from build123d import *

# Parameters (mm, degrees)
F0_R     = 2.5
F2_DEPTH = 492


with BuildPart() as f2:
    # F0 (on Front) → F2 (new body)
    with BuildSketch(Plane.XZ):
        with BuildLine():
            Line((6.5, 0), (2, 0))
            ThreePointArc((2, 0), (0.5857864376, -0.5857864376), (0, -2))
            Line((0, -2), (0, -6.4857100192))
            Line((0, -6.4857100192), (0.4948230833, -6.489995392))
            Line((0.4948230833, -6.489995392), (0.4948230833, -7))
            Line((0.4948230833, -7), (2, -7))
            Line((2, -7), (2, -3.0833937817))
            Line((2, -3.0833937817), (6.2, -7.2637052917))
            Line((6.2, -7.2637052917), (6.2, -12.7393398282))
            Line((6.2, -12.7393398282), (2, -16.9393398282))
            Line((2, -16.9393398282), (2, -13))
            Line((2, -13), (0.5, -13))
            Line((0.5, -13), (0.5, -13.5))
            Line((0.5, -13.5), (0, -13.5))
            Line((0, -13.5), (0, -26.4857100192))
            Line((0, -26.4857100192), (0.4948230833, -26.489995392))
            Line((0.4948230833, -26.489995392), (0.4948230833, -27))
            Line((0.4948230833, -27), (2, -27))
            Line((2, -27), (2, -23.0833937817))
            Line((2, -23.0833937817), (6.2, -27.2637052917))
            Line((6.2, -27.2637052917), (6.2, -32.7393398282))
            Line((6.2, -32.7393398282), (2, -36.9393398282))
            Line((2, -36.9393398282), (2, -33))
            Line((2, -33), (0.5, -33))
            Line((0.5, -33), (0.5, -33.5))
            Line((0.5, -33.5), (0, -33.5))
            Line((0, -33.5), (0, -38))
            ThreePointArc((0, -38), (0.5857864376, -39.4142135624), (2, -40))
            Line((2, -40), (6.5, -40))
            Line((6.5, -40), (6.5, -39.5))
            Line((6.5, -39.5), (7, -39.5))
            Line((7, -39.5), (7, -38))
            Line((7, -38), (3.0606601718, -38))
            Line((3.0606601718, -38), (7.2606601718, -33.8))
            Line((7.2606601718, -33.8), (12.7393398282, -33.8))
            Line((12.7393398282, -33.8), (16.9393398282, -38))
            Line((16.9393398282, -38), (13.015800612, -38))
            Line((13.015800612, -38), (13.015800612, -39.5))
            Line((13.015800612, -39.5), (13.5, -39.5))
            Line((13.5, -39.5), (13.5, -40))
            Line((13.5, -40), (18, -40))
            ThreePointArc((18, -40), (19.4142135624, -39.4142135624), (20, -38))
            Line((20, -38), (20, -33.4626608249))
            Line((20, -33.4626608249), (19.5363645284, -33.4624647606))
            Line((19.5363645284, -33.4624647606), (19.532302618, -32.9822008219))
            Line((19.532302618, -32.9822008219), (18, -32.9822008219))
            Line((18, -32.9822008219), (17.9998106987, -36.9393398192))
            Line((17.9998106987, -36.9393398192), (13.8264202785, -32.765949399))
            Line((13.8264202785, -32.765949399), (13.8264202785, -27.246708479))
            Line((13.8264202785, -27.246708479), (17.9998106987, -23.0606601627))
            Line((17.9998106987, -23.0606601627), (17.9998106987, -26.9999999909))
            Line((17.9998106987, -26.9999999909), (19.4998106987, -26.9999999909))
            Line((19.4998106987, -26.9999999909), (19.4998106987, -26.4999999909))
            Line((19.4998106987, -26.4999999909), (20, -26.4999999909))
            Line((20, -26.4999999909), (20, -13.4626608249))
            Line((20, -13.4626608249), (19.5363645284, -13.4624647606))
            Line((19.5363645284, -13.4624647606), (19.532302618, -12.9822008219))
            Line((19.532302618, -12.9822008219), (18, -12.9822008219))
            Line((18, -12.9822008219), (17.9998106987, -16.9393398192))
            Line((17.9998106987, -16.9393398192), (13.8264202785, -12.765949399))
            Line((13.8264202785, -12.765949399), (13.8264202785, -7.246708479))
            Line((13.8264202785, -7.246708479), (17.9998106987, -3.0606601627))
            Line((17.9998106987, -3.0606601627), (17.9998106987, -6.9999999909))
            Line((17.9998106987, -6.9999999909), (19.4998106987, -6.9999999909))
            Line((19.4998106987, -6.9999999909), (19.4998106987, -6.4999999909))
            Line((19.4998106987, -6.4999999909), (20, -6.4999999909))
            Line((20, -6.4999999909), (20, -2))
            ThreePointArc((20, -2), (19.4142135624, -0.5857864376), (18, 0))
            Line((18, 0), (13.4962801728, 0.0202495232))
            Line((13.4962801728, 0.0202495232), (13.5, -0.5))
            Line((13.5, -0.5), (13.015800612, -0.5))
            Line((13.015800612, -0.5), (13.015800612, -2))
            Line((13.015800612, -2), (16.9393398282, -2))
            Line((16.9393398282, -2), (12.7393121854, -6.2000276428))
            Line((12.7393121854, -6.2000276428), (7.2606601718, -6.2))
            Line((7.2606601718, -6.2), (3.0606601718, -2))
            Line((3.0606601718, -2), (7, -2))
            Line((7, -2), (7, -0.5))
            Line((7, -0.5), (6.5, -0.5))
            Line((6.5, -0.5), (6.5, 0))
        make_face()
        with Locations((10, -30)):
            Circle(F0_R, mode=Mode.SUBTRACT)
        Polygon((7.2606601718, -13.8), (12.7393398282, -13.8), (16.9393398282, -18), (16.9393398282, -22), (12.7393121854, -26.2000276428), (7.2606601718, -26.2), (3.0606601718, -22), (3.0606601718, -18), align=None, mode=Mode.SUBTRACT)
        with Locations((10, -10)):
            Circle(F0_R, mode=Mode.SUBTRACT)
    extrude(amount=F2_DEPTH)


solid = f2.part
For this review, take the finished solid that the model builds, in its own axes (mm). Give positions to 0.01 mm unless a question says otherwise; leave off trailing zeros. Put each result on its own line as item: value. Start each with the question number.
(1) Wall thickness on L1, parallel to Z at x = 10, y = -223; L2, parallel to Z at x = 1.5, y = -55.5; L3, parallel to Z at x = 14.75, y = -121.5: over which ranges is each line inside the solid? List them lowest first.
(2) Add section A-A, the plane y = -281. Give the number of separate pieces and of enclosed holes in the cut face, then the cut area to 3 significant figures.
(3) For pin 1 (8 mm diameter, centred on y = -365, z = -25.5, fed in from -X); pin 2 (4 mm diameter, centred on x = 6.5, z = -20.5, fed in from +Y); pin 3 (0.5 mm diameter, centred on x = 13, y = -358.5, fed in from -Z); pin 4 (4.5 mm diameter, centred on y = -295.5, z = -29, fed in from +X), all flat-tipped, find the tip position at first contact; note any pin that passes through.
Result:
1. L1: z = -33.8 to -32.5, -27.5 to -26.2, -13.8 to -12.5, -7.5 to -6.2
1. L2: z = -39.94 to -33, -27 to -13, -7 to -0.06
1. L3: z = -40 to -38, -35.81 to -33.69, -26.32 to -24.19, -15.81 to -13.69, -6.32 to -4.19, -2 to 0.01
2. separate pieces: 1
2. enclosed holes: 3
2. area: 302 mm^2
3. pin 1: stops at x = 0
3. pin 2: passes through
3. pin 3: stops at z = -39.5
3. pin 4: stops at x = 19.5
